Autodesk Inventor part; units mm, degrees
ref_plane "作業平面2" through (0, 76.6523, 179.1954) normal (0, 1, 0) x (1, 0, 0)
ref_plane "YZ Plane" through (0, 0, 0) normal (1, 0, 0) x (0, 1, 0)
ref_plane "XZ Plane" through (0, 0, 0) normal (0, 1, 0) x (-1, 0, 0)
sketch "スケッチ1" plane through (0, 0, 0) normal (1, 0, 0) x (0, 1, 0)
  line L0 (125.6523, 179.1954) -> (-474.3477, 179.1954)
  line L1 (-474.3477, 179.1954) -> (-474.3477, -102.8046)
  line L2 (-474.3477, -102.8046) -> (125.6523, -102.8046)
  line L3 (125.6523, -102.8046) -> (125.6523, 179.1954)
  dimension "d0" = 600
  dimension "d1" = 282
extrude "押し出し1" add sketch "スケッチ1" along normal blind 2.6
sketch "スケッチ4" plane through (2.6, 0, 0) normal (1, 0, 0) x (0, 0, -1)
  line L0 (102.8046, 125.6523) -> (-179.1954, 125.6523)
  line L1 (-179.1954, 125.6523) -> (-179.1954, -474.3477)
  point P0 (0, 0)
  point P1 (-139.1954, -225.3477)
  point P2 (-139.1954, -123.3477)
  dimension "d19" = 102
  dimension "d20" = 249
  dimension "d21" = 40
  dimension "d22" = 40
hole "穴2" at (2.6, -225.3477, 139.1954) at (2.6, -123.3477, 139.1954) direction (-1, 0, 0) diameter 6.6 end through all
sketch "スケッチ5" plane through (2.6, 0, 0) normal (1, 0, 0) x (0, 0, -1)
  line L0 (-179.1954, 125.6523) -> (-179.1954, -474.3477)
  line L1 (102.8046, 125.6523) -> (-179.1954, 125.6523)
  point P0 (-152.1954, -84.3477)
  dimension "d30" = 27
  dimension "d31" = 210
hole "穴3" at (2.6, -84.3477, 152.1954) direction (-1, 0, 0) diameter 18 end through all
sketch "スケッチ6" plane through (2.6, 0, 0) normal (1, 0, 0) x (0, 0, -1)
  line L0 (-179.1954, 125.6523) -> (-179.1954, -474.3477)
  circle A0 centre (-152.1954, -84.3477) radius 9
  point P0 (0, 0)
  point P1 (-166.6954, -53.9477)
  point P2 (-151.6954, -53.9477)
  dimension "d39" = 12.5
  dimension "d40" = 27.5
  dimension "d41" = 30.4
  dimension "d42" = 30.4
hole "穴4" at (2.6, -53.9477, 166.6954) at (2.6, -53.9477, 151.6954) direction (-1, 0, 0) diameter 4.5 end through all
sketch "スケッチ7" plane through (2.6, 0, 0) normal (1, 0, 0) x (0, 0, -1)
  line L0 (102.8046, 125.6523) -> (-179.1954, 125.6523)
  line L1 (102.8046, -474.3477) -> (102.8046, 125.6523)
  line L2 (-179.1954, -474.3477) -> (102.8046, -474.3477)
  point P0 (0, 0)
  point P1 (84.0046, -56.9477)
  point P2 (84.0046, -291.9477)
  dimension "d50" = 182.6
  dimension "d51" = 18.8
  dimension "d52" = 18.8
  dimension "d53" = 182.4
hole "穴5" at (2.6, -56.9477, -84.0046) at (2.6, -291.9477, -84.0046) direction (-1, 0, 0) diameter 6.7 end through all
sketch "スケッチ8" plane through (2.6, 0, 0) normal (1, 0, 0) x (0, 0, -1)
  line L0 (102.8046, -474.3477) -> (102.8046, 125.6523)
  line L1 (102.8046, 125.6523) -> (110.8046, 125.6523)
  line L2 (117.7603, -23.9477) -> (102.8046, -23.9477)
  line L3 (102.8046, -89.9477) -> (117.7603, -89.9477)
  line L4 (110.8046, 125.6523) -> (110.8046, -474.3477)
  line L5 (110.8046, -474.3477) -> (102.8046, -474.3477)
  line L6 (102.8046, -258.9477) -> (110.8046, -258.9477)
  line L7 (102.8046, -324.9477) -> (110.8046, -324.9477)
  circle A0 centre (84.0046, -56.9477) radius 3.35
  circle A1 centre (84.0046, -291.9477) radius 3.35
  point P0 (0, 0)
  point P1 (110.8046, -23.9477)
  point P2 (110.8046, -89.9477)
  dimension "d61" = 8
  dimension "d62" = 33
  dimension "d63" = 33
  dimension "d64" = 33
  dimension "d65" = 33
extrude "押し出し3" add sketch "スケッチ8" against normal blind 2.6 contours L0 L7 L4 L5 | L0 L3 L4 L6 | L0 L1 L4 L2
sketch "スケッチ9" plane through (2.6, 0, 0) normal (1, 0, 0) x (0, 0, -1)
  ellipse E0 centre (-2.4593, 110.6523) end of major axis (-2.4593, 125.1521) minor radius 14.4996 (5.606, 98.6026) -> (5.606, 122.702) ccw
  line L0 (4.4935, 123.5363) -> (-99.9579, 123.5363)
  line L1 (-99.9579, 97.7683) -> (4.4935, 97.7683)
  ellipse E1 centre (-67.383, 110.6523) end of major axis (-67.383, 123.067) minor radius 12.4145 (-70.683, 122.6204) -> (-70.683, 98.6842) ccw
  line L2 (-70.683, 122.6204) -> (-70.683, 125.6523)
  line L3 (102.8046, 125.6523) -> (-179.1954, 125.6523)
  line L4 (5.7266, 122.6204) -> (5.7266, 125.6523)
  line L5 (5.7266, 125.6523) -> (-70.683, 125.6523)
  line L6 (6.1243, 98.9661) -> (4.4935, 97.7683)
  line L7 (-70.683, 98.6842) -> (-66.6998, 97.7683)
  point P0 (0, 0)
extrude "押し出し4" cut sketch "スケッチ9" against normal blind 3
ref_plane "作業平面2" through (0, 76.6523, 179.1954) normal (0, 1, 0) x (1, 0, 0)
split "分割2" plane through (0, 76.6523, 179.1954) removes the side toward (0, -1, 0)
sketch "スケッチ10" plane through (2.6, 0, 0) normal (1, 0, 0) x (0, 0, -1)
  line L0 (-70.683, 125.6523) -> (-179.1954, 125.6523)
  line L1 (-179.1954, 125.6523) -> (-179.1954, 76.6523)
  line L2 (110.8046, 125.6523) -> (5.7266, 125.6523)
  line L3 (110.8046, 76.6523) -> (110.8046, 125.6523)
  point P0 (0, 0)
  point P1 (-169.1954, 115.6523)
  point P2 (100.8046, 115.6523)
  dimension "d72" = 10
  dimension "d73" = 10
  dimension "d74" = 10
  dimension "d75" = 10
hole "穴6" at (2.6, 115.6523, 169.1954) at (2.6, 115.6523, -100.8046) direction (-1, 0, 0) diameter 4.5 depth 6 tip angle 118
properties part number "lc_box_side" material "ポリカーボネート、クリア"
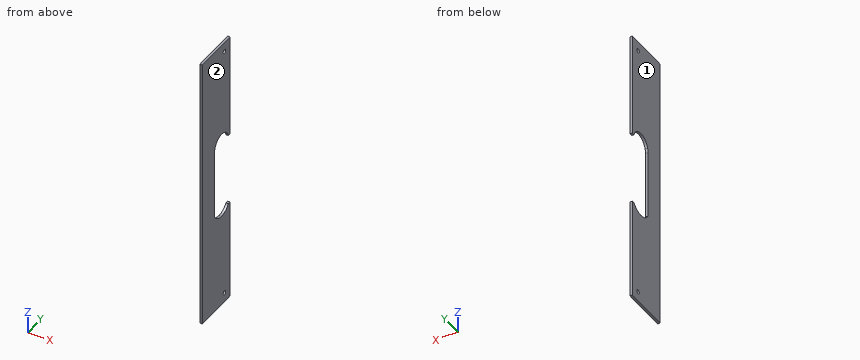
Work out the finished part from the listing and answer in its coordinate system (mm). Face numbers are marked on the shaded views. Round coordinates to 2 decimals unless told otherwise and drop trailing zeros. Write each loop counter-clockwise with the first axis right and the second up, starting at its lowest first coordinate (ties: lowest second). Pieces come first, ordered by that corner, then holes.
1) Consider probe 1 along Z at (x, y) = (2.05, 110); probe 2 along Z at (x, y) = (2.45, 114); probe 3 along Z at (x, y) = (1.25, 117.5). Determine where each line is inside the solid, lowest interval first.
2) Determine the mould class of the marked faces 1 and 2 for opening direction X: pulls with the +X half, pulls with the -X half, needs draft (parallel to the pull), parting line crosses it, or undercut.
3) A cutting plane is placed at B-B on x = 0.6. Give the number of separate pieces and of enclosed holes in the cut face, and give its area (3 significant figures).
4) A cutting plane is placed at A-A on z = 58.5. Determine the outline of the cut face in (x, y), and give its area (3 significant figures).
5) Flat-ended cylindrical pins translate along their axes: P1, Ø4, axis at y = 115.65, z = 169.2, coming from the +X side; P2, Ø1.3, axis at x = 1.5, z = 34.5, coming from the +Y side. Find the tip coordinate at first contact, or state that the pin passes through.
Entries:
1. probe 1: z = -110.8 to -12.03, 79.78 to 179.2
1. probe 2: z = -110.8 to -102.33, -99.28 to -11.65, 79.34 to 167.67, 170.72 to 179.2
1. probe 3: z = -110.8 to -102.09, -99.52 to -10.32, 77.74 to 167.91, 170.48 to 179.2
2. face 1: pulls with the -X half
2. face 2: pulls with the +X half
3. separate pieces: 1
3. enclosed holes: 2
3. area: 11,800 mm2
4. outline: (0, 76.65) - (2.6, 76.65) - (2.6, 97.77) - (0, 97.77) - close
4. area: 54.9 mm2
5. P1: passes through
5. P2: stops at y = 97.77
